from build123d import *

# Parameters (mm, degrees)
F0_R     = 1.5
F0_R_2   = 3
F1_DEPTH = 2
F2_R     = 6
F2_R_2   = 3
F3_DEPTH = 2
F4_R     = 1.49999
F5_SIZE  = 1
F6_SIZE  = 0.49999


# Not quite as in the source:
# - a fillet or chamfer is up to 0.001 mm smaller than in the source, because OpenCascade refuses the exact size


with BuildPart() as f1:
    # F0 (on Top) → F1 (new body)
    with BuildSketch(Plane.XY):
        Polygon((-6, 3), (-13, 3), (-13, -3), (-6, -3), (-6, -6), (6, -6), (6, -3), (13, -3), (13, 3), (6, 3), (6, 6), (-6, 6), align=None)
        with Locations((-8, 0)):
            Circle(F0_R, mode=Mode.SUBTRACT)
        Circle(F0_R_2, mode=Mode.SUBTRACT)
        with Locations((8, 0)):
            Circle(F0_R, mode=Mode.SUBTRACT)
    extrude(amount=F1_DEPTH)

    # F2 (on face) → F3 (join)
    with BuildSketch(Plane.XY.offset(2)):
        Circle(F2_R)
        Circle(F2_R_2, mode=Mode.SUBTRACT)
    extrude(amount=F3_DEPTH)

    # F4 (radius 1.5 in the source; OpenCascade refuses exactly that, so slightly less here)
    f4_edges = [f1.edges().sort_by_distance(p)[0] for p in [
        (-6, -6, 1),
        (6, -6, 1),
        (6, 6, 1),
        (-6, 6, 1),
        (-6, 3, 1),
        (-6, -3, 1),
        (6, 3, 1),
        (6, -3, 1),
    ]]
    fillet(f4_edges, radius=F4_R)

    # F5
    f5_edges = [f1.edges().sort_by_distance(p)[0] for p in [
        (-3, 0, 0),
    ]]
    chamfer(f5_edges, length=F5_SIZE)

    # F6 (size 0.5 in the source; OpenCascade refuses exactly that, so slightly less here)
    f6_edges = [f1.edges().sort_by_distance(p)[0] for p in [
        (-9.5, 0, 2),
        (6.5, 0, 2),
    ]]
    chamfer(f6_edges, length=F6_SIZE)


solid = f1.part
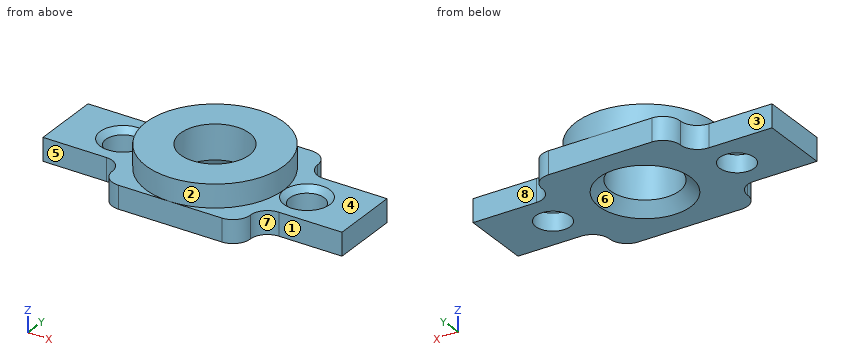
For this review, take the finished solid that the model builds, in its own axes (mm). Face numbers are marked on the shaded views. A direction names the side the tool comes from. Round coordinates to 2 decimals unless told otherwise and drop trailing zeros. Write each loop counter-clockwise with the first axis right and the second up, starting at its lowest first coordinate (ties: lowest second). Pieces come first, ordered by that corner, then holes. Notation, with made-up numbers: (87, 65) - (98, 65) arc R19 ccw to (98, 90) - close; hole circle Ø5 at (-15.75, -18). An arc over 180 degrees is marked (long way). Use a Markdown table: item, result.
Q1. We need section D-D (z = 3.05). Give the boundary of the cut face in (x, y).
Derived:
| item | result |
|---|---|
| outline | circle Ø12 at (0, 0); hole circle Ø6 at (0, 0) |
Q2. The part is to be moulded in two halves that separate along Y. For the marked faces 6, 7 and 8, say which applies: pulls with the +Y half, pulls with the -Y half, needs draft (parallel to the pull), parting line crosses it, or undercut.
Derived:
| item | result |
|---|---|
| face 6 | undercut |
| face 7 | pulls with the -Y half |
| face 8 | pulls with the +Y half |
Q3. We need section B-B (x = 8). Give the boundary of the cut face in (y, z), plus the area to 3 significant figures.
Derived:
| item | result |
|---|---|
| outline | (-3, 0) - (-1.5, 0) - (-1.5, 1.5) - (-2, 2) - (-3, 2) - close; (1.5, 0) - (3, 0) - (3, 2) - (2, 2) - (1.5, 1.5) - close |
| area | 5.75 mm2 |
Q4. Wall thickness on line 1 along Y through (x, z) = (8, 1); line 2 along Y through (x, z) = (0, 1.95); line 3 along Z through (x, y) = (10.5, -0.75): over which ranges is each line inside the solid? List them lowest first.
Derived:
| item | result |
|---|---|
| line 1 | y = -3 to -1.5, 1.5 to 3 |
| line 2 | y = -6 to -3, 3 to 6 |
| line 3 | z = 0 to 2 |
Q5. Clearance check with flat-ended pins moving along their axes: pin 1 (3 mm diameter, centred on x = 1, y = 1, fed in from -Z); pin 2 (1 mm diameter, centred on x = -11, z = 1, fed in from +Y); pin 3 (1.6 mm diameter, centred on x = -11.5, z = 0.5, fed in from -Y); pin 4 (3.5 mm diameter, centred on x = -9, y = -2.5, fed in from +Z). State where each tip first meets the part, or that it passes through.
Derived:
| item | result |
|---|---|
| pin 1 | passes through |
| pin 2 | stops at y = 3 |
| pin 3 | stops at y = -3 |
| pin 4 | stops at z = 2 |
Q6. Machinability: for the marked faces 1, 2, 3, 4 and 5, which of the approach directions +Z, -Z, +X, -X, +Y, -Y give a long, thin tool a straight path to every point of the face, cutting with its end or side? Answer none if there is none.
Derived:
| item | result |
|---|---|
| face 1 | +Z, -Z, +X, -Y |
| face 2 | +Z |
| face 3 | +Z, -Z, -X, +Y |
| face 4 | +Z, +X |
| face 5 | +Z, -Z, -X, -Y |
Q7. We need section A-A (y = 0). State how many separate pieces and enclosed holes the cut face has, plus the area to 3 significant figures.
Derived:
| item | result |
|---|---|
| separate pieces | 4 |
| enclosed holes | 0 |
| area | 38.5 mm2 |
